```python
from build123d import *

# Parameters (mm, degrees)
PLACA_ANTEBRAZO_START          = -3.175
PLACA_ANTEBRAZO_DEPTH          = 6.35
PLACA_ANTEBRAZO_REDONDEO_START = -3.175
CROQUIS13_R                    = 25
PLACA_ANTEBRAZO_REDONDEO_DEPTH = 6.35
BARRENOS_J3_START              = -3.175
CROQUIS14_R                    = 1.7
CROQUIS14_R_2                  = 2.05
CROQUIS14_R_3                  = 3.4
BARRENOS_J3_DEPTH              = 6.35
REFRENTADOS_J3_START           = -3.175
CROQUIS15_R                    = 3
REFRENTADOS_J3_DEPTH           = 3.2
ALIGERADO_PASO_CABLE_START     = -3.175
ALIGERADO_PASO_CABLE_DEPTH     = 6.35
ROSCA_M3_CANTO_START           = 213.25
CROQUIS17_R                    = 1.25
ROSCA_M3_CANTO_DEPTH           = 9
PASADORES_D3_START             = 215.25
CROQUIS18_R                    = 1.5
PASADORES_D3_DEPTH             = 7
PASO_M3_BASES_CINCHO_START     = -3.175
CROQUIS20_R                    = 1.7
PASO_M3_BASES_CINCHO_DEPTH     = 6.35
CROQUIS21_R                    = 7.45
CORTAR_EXTRUIR1_DEPTH          = 5


with BuildPart() as part:
    # Croquis12 → Placa_antebrazo (new body)
    with BuildSketch(Plane(origin=(0, 0, 0), x_dir=(1, 0, 0), z_dir=(0, 1, 0)).offset(PLACA_ANTEBRAZO_START)):
        Polygon((127.4, -171.45), (177.4, -171.45), (182.4, -222.25), (122.4, -222.25), align=None)
    extrude(amount=PLACA_ANTEBRAZO_DEPTH)

    # Croquis13 → Placa_antebrazo_redondeo (add)
    with BuildSketch(Plane(origin=(0, 0, 0), x_dir=(1, 0, 0), z_dir=(0, 1, 0)).offset(PLACA_ANTEBRAZO_REDONDEO_START)):
        with Locations((152.4, -171.45)):
            Circle(CROQUIS13_R)
    extrude(amount=PLACA_ANTEBRAZO_REDONDEO_DEPTH)

    # Croquis14 → Barrenos_J3 (cut)
    with BuildSketch(Plane(origin=(0, 0, 0), x_dir=(1, 0, 0), z_dir=(0, 1, 0)).offset(BARRENOS_J3_START)):
        with Locations(Location((163.416293151, -177.356884561, 0), (0, 0, 270))):
            Circle(CROQUIS14_R)
        with Locations(Location((152.792634488, -183.943832005, 0), (0, 0, 270))):
            Circle(CROQUIS14_R)
        with Locations(Location((141.776341338, -178.036947444, 0), (0, 0, 270))):
            Circle(CROQUIS14_R)
        with Locations(Location((141.383706849, -165.543115439, 0), (0, 0, 270))):
            Circle(CROQUIS14_R)
        with Locations(Location((152.007365512, -158.956167995, 0), (0, 0, 270))):
            Circle(CROQUIS14_R)
        with Locations(Location((163.023658662, -164.863052556, 0), (0, 0, 270))):
            Circle(CROQUIS14_R)
        with Locations(Location((157.774949114, -180.118905468, 0), (0, 0, 270))):
            Circle(CROQUIS14_R_2)
        with Locations(Location((142.205033084, -171.770389743, 0), (0, 0, 270))):
            Circle(CROQUIS14_R_2)
        with Locations(Location((157.220017802, -162.460704789, 0), (0, 0, 270))):
            Circle(CROQUIS14_R_2)
        with Locations(Location((152.4, -171.45, 0), (0, 0, 270))):
            Circle(CROQUIS14_R_3)
    extrude(amount=BARRENOS_J3_DEPTH, mode=Mode.SUBTRACT)

    # Croquis15 → Refrentados_J3 (cut)
    with BuildSketch(Plane(origin=(0, 0, 0), x_dir=(1, 0, 0), z_dir=(0, 1, 0)).offset(REFRENTADOS_J3_START)):
        with Locations(Location((163.416293151, -177.356884561, 0), (0, 0, 90))):
            Circle(CROQUIS15_R)
        with Locations(Location((152.792634488, -183.943832005, 0), (0, 0, 90))):
            Circle(CROQUIS15_R)
        with Locations(Location((141.776341338, -178.036947444, 0), (0, 0, 90))):
            Circle(CROQUIS15_R)
        with Locations(Location((141.383706849, -165.543115439, 0), (0, 0, 90))):
            Circle(CROQUIS15_R)
        with Locations(Location((152.007365512, -158.956167995, 0), (0, 0, 90))):
            Circle(CROQUIS15_R)
        with Locations(Location((163.023658662, -164.863052556, 0), (0, 0, 90))):
            Circle(CROQUIS15_R)
    extrude(amount=REFRENTADOS_J3_DEPTH, mode=Mode.SUBTRACT)

    # Croquis16 → Aligerado_paso_cable (cut)
    with BuildSketch(Plane(origin=(0, 0, 0), x_dir=(1, 0, 0), z_dir=(0, 1, 0)).offset(ALIGERADO_PASO_CABLE_START)):
        with BuildLine():
            Line((158.4, -195), (158.4, -210))
            ThreePointArc((158.4, -210), (152.4, -216), (146.4, -210))
            Line((146.4, -210), (146.4, -195))
            ThreePointArc((146.4, -195), (152.4, -189), (158.4, -195))
        make_face()
    extrude(amount=ALIGERADO_PASO_CABLE_DEPTH, mode=Mode.SUBTRACT)

    # Croquis17 → Rosca_M3_canto (cut)
    with BuildSketch(Plane.XY.offset(ROSCA_M3_CANTO_START)):
        with Locations((125.4, 0)):
            Circle(CROQUIS17_R)
        with Locations((179.4, 0)):
            Circle(CROQUIS17_R)
    extrude(amount=ROSCA_M3_CANTO_DEPTH, mode=Mode.SUBTRACT)

    # Croquis18 → Pasadores_D3 (cut)
    with BuildSketch(Plane.XY.offset(PASADORES_D3_START)):
        with Locations((138.4, 0)):
            Circle(CROQUIS18_R)
        with Locations((166.4, 0)):
            Circle(CROQUIS18_R)
    extrude(amount=PASADORES_D3_DEPTH, mode=Mode.SUBTRACT)

    # Croquis20 → Paso_M3_bases_cincho (cut)
    with BuildSketch(Plane(origin=(0, 0, 0), x_dir=(1, 0, 0), z_dir=(0, 1, 0)).offset(PASO_M3_BASES_CINCHO_START)):
        with Locations(Location((168.9, -211, 0), (0, 0, 270))):
            Circle(CROQUIS20_R)
    extrude(amount=PASO_M3_BASES_CINCHO_DEPTH, mode=Mode.SUBTRACT)

    # Croquis21 → Cortar-Extruir1 (cut)
    with BuildSketch(Plane.XZ.offset(3.175)):
        with Locations(Location((152.4, 171.45, 0), (0, 0, 270))):
            Circle(CROQUIS21_R)
    extrude(amount=-CORTAR_EXTRUIR1_DEPTH, mode=Mode.SUBTRACT)


solid = part.part
```
Could you check a few things on this model? Use its own coordinates, in mm. A direction names the side the tool comes from. Coordinates: 2 decimals unless noted, no trailing zeros. Write each loop counter-clockwise with the first axis right and the second up, starting at its lowest first coordinate (ties: lowest second). Pieces come first, ordered by that corner, then holes. Notation, with made-up numbers: (18, 88.25) -> (59, 88.25) arc R19 ccw to (59, 110.25) -> close; hole circle Ø1 at (58.5, 38). An arc over 180 degrees is marked (long way). One line per question, with ' | ' between items. Start each with the question number.
1. Thinking about a two-plate mould opening in Z: for faces 4 (the face through (162.77, 1.58, 178.93)), 5 (the face through (159, -3.175, 192)), 6 (the face through (179.865, -0.044, 196.494)), 7 (the face through (143, 0.025, 164)), which applies, pulls with the +Z half, pulls with the -Z half, needs draft (parallel to the pull), parting line crosses it, or undercut?
2. Please list where these lines run through material, in increasing order: line 1 along Z through (x, y) = (154, -2); line 2 along X through (y, z) = (-0.75, 177.5); line 3 along X through (y, z) = (-0.25, 170.5).
3. If we section it at A-A (z = 190.5): Please give me the cut outline in (x, y) (3 decimals).
4. If we section it at B-B (x = 125.4): Please give me the cut outline in (y, z) (3 decimals), and give its area (3 significant figures).
5. If we section it at C-C (z = 211): Please give me the cut outline in (x, y) (3 decimals).
6. If we section it at D-D (x = 171.5): Please give me the cut outline in (y, z) (3 decimals).
7. For faces 1 (the face through (138, 0, 215.25)), 2 (the face through (170.333, -0.044, 211.914)), 3 (the face through (155.454, -1.597, 182.56)), which set-ups out of +Z, -Z, +X, -X, +Y, -Y let a thin tool reach every point of the face, with its end or its side?
8. Will these pins go through, and if not, where does the flat tip stop? P1, Ø1.8, axis at x = 163.5, z = 176.5, coming from the -Y side (3 decimals); P2, Ø4.5, axis at x = 153.5, z = 170, coming from the -Y side (3 decimals); P3, Ø1.2, axis at x = 179, y = 0, coming from the +Z side; P4, Ø3, axis at x = 168.9, z = 211, coming from the -Y side.
Return value:
1) face 4: undercut | face 5: needs draft | face 6: pulls with the -Z half | face 7: undercut
2) line 1: z = 146.5 to 156.71, 161.2 to 164.17, 178.73 to 181.2, 186.69 to 189.22, 215.78 to 222.25 | line 2: x = 126.8 to 138.82, 144.73 to 148.05, 156.75 to 160.42, 166.41 to 178 | line 3: x = 127.42 to 140.6, 143.81 to 145.01, 159.79 to 177.38
3) outline: (125.525, -3.175) -> (148.431, -3.175) -> (148.431, 3.175) -> (125.525, 3.175) -> close; (156.369, -3.175) -> (179.275, -3.175) -> (179.275, 3.175) -> (156.369, 3.175) -> close
4) outline: (-3.175, 191.77) -> (3.175, 191.77) -> (3.175, 222.25) -> (1.25, 222.25) -> (1.25, 213.25) -> (-1.25, 213.25) -> (-1.25, 222.25) -> (-3.175, 222.25) -> close | area: 171 mm²
5) outline: (123.507, -3.175) -> (146.484, -3.175) -> (146.484, 3.175) -> (123.507, 3.175) -> close; (158.316, -3.175) -> (167.2, -3.175) -> (167.2, 3.175) -> (158.316, 3.175) -> close; (170.6, -3.175) -> (181.293, -3.175) -> (181.293, 3.175) -> (170.6, 3.175) -> close
6) outline: (-3.175, 155.32) -> (3.175, 155.32) -> (3.175, 222.25) -> (-3.175, 222.25) -> close
7) face 1: +Z | face 2: +Y, -Y | face 3: -Y
8) P1: stops at y = 0.025 | P2: stops at y = 1.825 | P3: stops at z = 213.25 | P4: passes through
